```python
from build123d import *

# Parameters (mm, degrees)
F0_W     = 100
F0_H     = 75
F1_DEPTH = 10
F2_T     = -2
F3_W     = 88
F3_H     = 69
F4_DEPTH = 5
F6_DEPTH = 10.001


with BuildPart() as f1:
    # F0 (on Front) → F1 (new body)
    with BuildSketch(Plane.XZ):
        with Locations((-50, 37.5)):
            Rectangle(F0_W, F0_H)
    extrude(amount=F1_DEPTH)

    # F2
    f2_openings = [f1.faces().sort_by_distance(p)[0] for p in [
        (-50, -5, 75),
    ]]
    offset(amount=F2_T, openings=f2_openings)

    # F3 (on face) → F4 (cut)
    with BuildSketch(Plane.XZ.offset(10)):
        with Locations((-50, 40.5)):
            Rectangle(F3_W, F3_H)
    extrude(amount=-F4_DEPTH, mode=Mode.SUBTRACT)

    # F5 (on face) → F6 (cut, through all)
    with BuildSketch(Plane.XZ.offset(10)):
        with BuildLine():
            ThreePointArc((-56.115779, 75), (-52.745338, 62.328554), (-42, 69.842748))
            ThreePointArc((-42, 69.842748), (-42.485806, 72.588087), (-43.884221, 75))
            Line((-43.884221, 75), (-56.115779, 75))
        make_face()
    extrude(amount=-F6_DEPTH, mode=Mode.SUBTRACT)


solid = f1.part
```
Geometry check sheet. Reference: the model listing, model coordinates, mm. A direction names the side the tool comes from. Coordinates: 2 decimals unless noted, no trailing zeros. Write each loop counter-clockwise with the first axis right and the second up, starting at its lowest first coordinate (ties: lowest second). Pieces come first, ordered by that corner, then holes. Notation, with made-up numbers: M 37,44.5 L 61,44.5 A15 ccw 61,49.5 Z; hole C 12.25,50.25 d6. An arc over 180 degrees is marked long. One line per item, written item: value. Start each with the question number.
(1) Sectioned sample at B-B, the plane x = -65.5. Enter the section's corners in (y, z), and give its area (3 significant figures).
(2) Tool access check on faces 4 (the face through (-100, -5, 37)), 5 (the face through (-50, -8, 4)), 6 (the face through (-94, -9, 40)). Record the directions out of +Z, -Z, +X, -X, +Y, -Y that give a thin tool (end or side, any length) a straight path to the whole face; none if there is none.
(3) Sectioned sample at A-A, the plane z = 63.5. Enter the section's corners in (x, y).
(4) Sectioned sample at C-C, the plane y = -5.5. Enter the section's corners in (x, z), and give its area (3 significant figures).
(5) Release check for a two-part mould opening along Y. For faces 1 (the face through (-51, -9, 6)), 2 (the face through (-50, -10, 4)), 3 (the face through (-98, -5, 38)) record: released by +Y, released by -Y, zero draft, split by the parting line, or undercut.
(6) Depth check by flat-ended pin: pin 1 (2 mm diameter, centred on x = -59.5, y = -9.5, fed in from +Z); pin 2 (22 mm diameter, centred on x = -30, z = 53, fed in from -Y). Enter the tip coordinate at first touch or a pass-through.
(7) Scan lines: line 1 along X through (y, z) = (-7.5, 68); line 2 along X through (y, z) = (-8.5, 67); line 3 along Y through (x, z) = (-66, 70). Record each from-to range of solid material in increasing order. Write a range as [from, to].
(8) Sectioned sample at D-D, the plane z = 11.5. Enter the section's corners in (x, y).
Filled sheet:
1. outline: M -10,0 L 0,0 L 0,75 L -2,75 L -2,2 L -8,2 L -8,6 L -10,6 Z
1. area: 174 mm²
2. face 4: +Z, -Z, -X, +Y, -Y
2. face 5: +Z
2. face 6: +Z, -Y
3. outline: M -100,-10 L -94,-10 L -94,-8 L -98,-8 L -98,-2 L -54.88,-2 L -54.88,0 L -100,0 Z; M -45.12,-2 L -2,-2 L -2,-8 L -6,-8 L -6,-10 L 0,-10 L 0,0 L -45.12,0 Z
4. outline: M -100,0 L 0,0 L 0,75 L -2,75 L -2,2 L -98,2 L -98,75 L -100,75 Z
4. area: 492 mm²
5. face 1: zero draft
5. face 2: released by -Y
5. face 3: undercut
6. pin 1: z = 6
6. pin 2: y = -2
7. line 1: [-100, -98], [-2, 0]
7. line 2: [-100, -94], [-6, 0]
7. line 3: [-2, 0]
8. outline: M -100,-10 L -94,-10 L -94,-8 L -98,-8 L -98,-2 L -2,-2 L -2,-8 L -6,-8 L -6,-10 L 0,-10 L 0,0 L -100,0 Z
